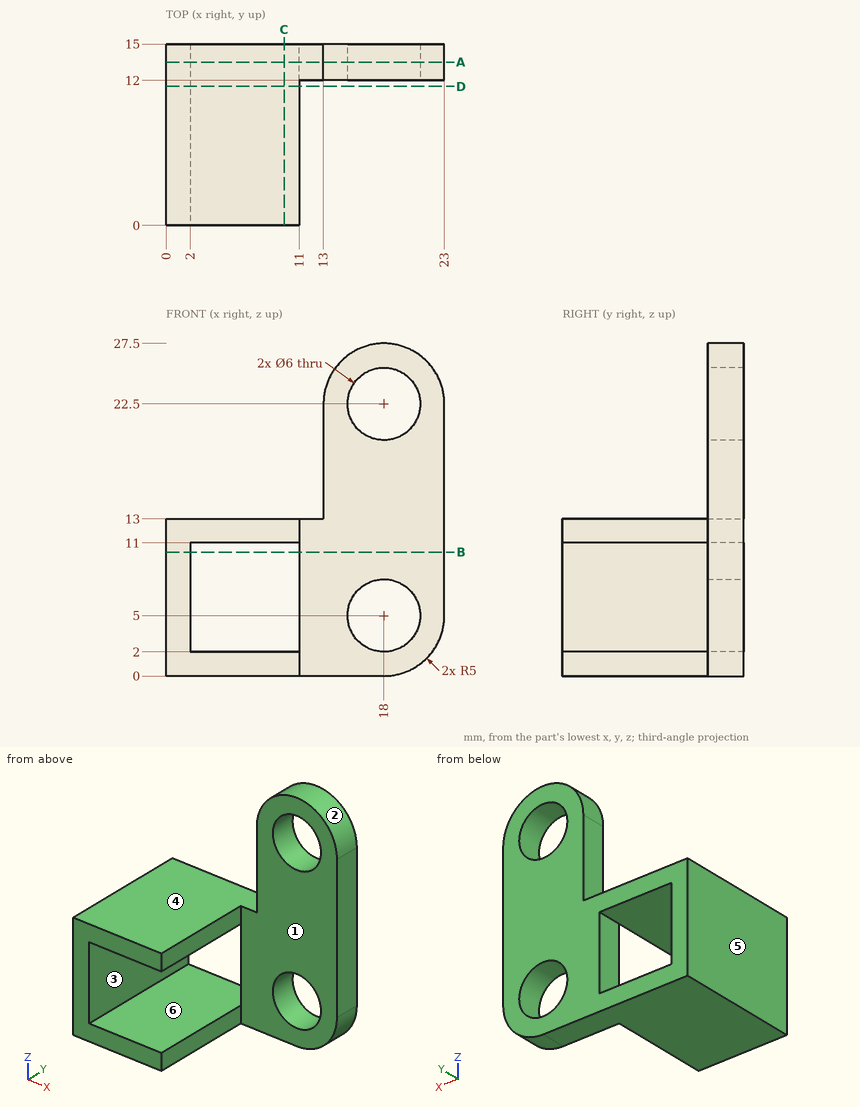
Could you check a few things on this drawing? It's one solid part, dimensions in mm from its lowest x, y, z. A direction names the side the tool comes from. Coordinates: 2 decimals unless noted, no trailing zeros. Loops run counter-clockwise (first coordinate to the right, second up) from the corner with the lowest first, then second, coordinate; pieces in that order, holes last. Notation, with made-up numbers: (-8, 56.5) - (37, 56.5) arc R27 ccw to (37, 76.5) - close; hole circle Ø3 at (34, 85). An arc over 180 degrees is marked (long way). Answer as a JSON object with one key per item and string values. Group by question number.
Item 1: If we section it at B-B (z = 10.25): List the corners of the cut face in (x, y) for me.
Item 2: If we section it at A-A (y = 13.5): List the corners of the cut face in (x, z) for me.
Item 3: If we section it at C-C (x = 9.75): List the corners of the cut face in (y, z) for me.
Item 4: On a 3-axis mill with a long thin cutter (end or side, diameter ignored), from which of +Z, -Z, +X, -X, +Y, -Y can I reach the whole of each face in a straight line? I mean the marked faces 4, 5 and 6. Say none if no direction works.
Item 5: If we mould it in two halves opening along X, with no side actions, what happens to the marked faces 1, 2 and 3? For each: released by +X, released by -X, zero draft, split by the parting line, or undercut.
Item 6: If we section it at D-D (y = 11.5): List the corners of the cut face in (x, z) for me.
Item 7: If I drill on L1, parallel to X at y = 13.7, z = 5; L2, parallel to Z at x = 18, y = 13; L3, parallel to Z at x = 7.5, y = 2, over which ranges is the centre line in solid material (lowest first)? Write a range as from..to.
Item 8: For pin 1 (3.5 mm diameter, centred on x = 20, z = 9, fed in from -Y); pin 2 (5 mm diameter, centred on y = 7, z = 16.5, fed in from -X); pin 3 (1.6 mm diameter, centred on y = 8.5, z = 1, fed in from +X); pin 4 (2.5 mm diameter, centred on y = 13, z = 17, fed in from -X), each with a flat end and sliding along its axis, tell me the tip position at first contact or that it passes through.
Returned:
{
 "1": {"outline": "(0, 0) - (2, 0) - (2, 15) - (0, 15) - close; (11, 12) - (23, 12) - (23, 15) - (11, 15) - close"},
 "2": {"outline": "(0, 0) - (18, 0) arc R5 ccw to (23, 5) - (23, 22.5) arc R5 ccw to (13, 22.5) - (13, 13) - (0, 13) - close; hole (2, 2) - (11, 2) - (11, 11) - (2, 11) - close; hole circle Ø6 at (18, 5); hole circle Ø6 at (18, 22.5)"},
 "3": {"outline": "(0, 0) - (15, 0) - (15, 2) - (0, 2) - close; (0, 11) - (15, 11) - (15, 13) - (0, 13) - close"},
 "4": {"face 4": "+Z, -X, +Y, -Y", "face 5": "+Z, -Z, -X, +Y, -Y", "face 6": "+Y, -Y"},
 "5": {"face 1": "zero draft", "face 2": "split by the parting line", "face 3": "undercut"},
 "6": {"outline": "(0, 0) - (11, 0) - (11, 2) - (2, 2) - (2, 11) - (11, 11) - (11, 13) - (0, 13) - close"},
 "7": {"L1": "x = 0..2, 11..15, 21..23", "L2": "z = 0..2, 8..19.5, 25.5..27.5", "L3": "z = 0..2, 11..13"},
 "8": {"pin 1": "stops at y = 12", "pin 2": "passes through", "pin 3": "stops at x = 11", "pin 4": "stops at x = 13"}
}
